```python
from build123d import *

# Parameters (mm, degrees)
F0_W     = 24
F0_H     = 4.9
F0_H_2   = 4.1
F1_DEPTH = 12
F2_DEPTH = 6
F3_DEPTH = 10
F4_SIZE2 = 11.99999
F4_SIZE  = 9.99999
F6_DEPTH = 24
F7_DEPTH = 4
F8_SIZE2 = 1
F8_SIZE  = 8


# Not quite as in the source:
# - a fillet or chamfer is up to 0.001 mm smaller than in the source, because OpenCascade refuses the exact size


with BuildPart() as f1:
    # F0 (on Top) → F1 (new body)
    with BuildSketch(Plane.XY):
        with Locations((-88, -2.45)):
            Rectangle(F0_W, F0_H)
        with Locations((-88, -6.95)):
            Rectangle(F0_W, F0_H_2)
        with Locations((-88, -11.05)):
            Rectangle(F0_W, F0_H_2)
        with Locations((-88, -15.55)):
            Rectangle(F0_W, F0_H)
    extrude(amount=F1_DEPTH)

    # F0 (on Top) → F2 (cut)
    with BuildSketch(Plane.XY):
        with Locations((-88, -6.95)):
            Rectangle(F0_W, F0_H_2)
        with Locations((-88, -11.05)):
            Rectangle(F0_W, F0_H_2)
    extrude(amount=F2_DEPTH, mode=Mode.SUBTRACT)

    # F3 (add): a face of the model
    f3_faces = [f1.faces().sort_by_distance(p)[0] for p in [
        (-88, 0, 6),
    ]]
    extrude(f3_faces, amount=F3_DEPTH)

    # F4 (size 10 and 12 in the source; OpenCascade refuses exactly that, so slightly less here)
    f4_edges = [f1.edges().sort_by_distance(p)[0] for p in [
        (-88, 10, 0),
    ]]
    f4_side = f1.faces().sort_by_distance((-88, 2.55, 0))[0]
    chamfer(f4_edges, length=F4_SIZE, length2=F4_SIZE2, reference=f4_side)

    # F5 (on face) → F6 (join, through all)
    with BuildSketch(Plane.YZ.offset(-76)):
        Polygon((-13.1, 0), (-12.1, 0), (-13.1, 6), align=None)
    extrude(amount=-F6_DEPTH)

    # F7 (add): a face of the model
    f7_faces = [f1.faces().sort_by_distance(p)[0] for p in [
        (-88, -2.449995, 0),
    ]]
    extrude(f7_faces, amount=F7_DEPTH)

    # F8
    f8_edges = [f1.edges().sort_by_distance(p)[0] for p in [
        (-88, -4.9, -4),
    ]]
    f8_side = f1.faces().sort_by_distance((-88, -4.9, 1))[0]
    chamfer(f8_edges, length=F8_SIZE, length2=F8_SIZE2, reference=f8_side)


solid = f1.part
```
The model under review builds one solid part; all positions refer to its coordinate system, in mm. A direction names the side the tool comes from. Round coordinates to 2 decimals unless told otherwise and drop trailing zeros. Loops run counter-clockwise (first coordinate to the right, second up) from the corner with the lowest first, then second, coordinate; pieces in that order, holes last. Notation, with made-up numbers: (34.25, 88) - (56.25, 88) arc R19 cw to (56.25, 109) - close; hole circle Ø11 at (23, 23). An arc over 180 degrees is marked (long way). Write each question's results on one line, items separated by ' | '. Start each with the question number.
Q1. Take a section at C-C on z = 10.5. Give the boundary of the cut face in (x, y), plus the area to 3 significant figures.
Q2. Wall thickness on line 1 along Y through (x, z) = (-83, 1) (3 decimals); line 2 along Z through (x, y) = (-97, -7.25); line 3 along Y through (x, z) = (-91.75, 3.25): over which ranges is each line inside the solid? List them lowest first. Write a range as [from, to].
Q3. Tool access review of faces 4 (the flat face through (-100, -4, 6)), 5 (the flat face through (-88.168, -4.393, -0.056)), 6 (the flat face through (-88, 0, -2)), 7 (the flat face through (-76, -4, 6)), 8 (the flat face through (-88, -15, 0)): name each direction out of +Z, -Z, +X, -X, +Y, -Y from which nothing blocks a thin tool from reaching the whole face with its end or side.
Q4. Take a section at B-B on z = 2.5. Give the boundary of the cut face in (x, y).
Q5. Draft analysis for pull direction Y (two halves, no side actions). For faces 1 (the flat face through (-87.8, -12.6, 3)), 2 (the flat face through (-88, -18, 6)), 3 (the flat face through (-88, -4, 12)), state which applies: pulls with the +Y half, pulls with the -Y half, needs draft (parallel to the pull), parting line crosses it, or undercut.
Q6. Take a section at D-D on y = -9. Give the boundary of the cut face in (x, z), plus the area to 3 significant figures.
Q7. Insertion check: P1, Ø4, axis at x = -91.5, y = -10.5, coming from the -Z side; P2, Ø1.5, axis at x = -95.5, y = 5, coming from the -Z side; P3, Ø2, axis at x = -90, z = 2.5, coming from the +Y side; P4, Ø3, axis at y = -6.5, z = -1, coming from the -X side. Each pin has a flat end and moves straight along its axis. Give the tip position at first contact, or say it passes through.
Data:
1) outline: (-100, -18) - (-76, -18) - (-76, 8.75) - (-100, 8.75) - close | area: 642 mm²
2) line 1: y = [-18, -12.267], [-4.525, 0.833] | line 2: z = [6, 12] | line 3: y = [-18, -12.64], [-4.81, 2.71]
3) face 4: +Z, -Z, -X, +Y, -Y | face 5: -Z, +X, -X | face 6: -Z, +X, -X, +Y | face 7: +Z, -Z, +X, +Y, -Y | face 8: -Z, +X, -X, -Y
4) outline: (-100, -18) - (-76, -18) - (-76, -12.52) - (-100, -12.52) - close; (-100, -4.71) - (-76, -4.71) - (-76, 2.08) - (-100, 2.08) - close
5) face 1: undercut | face 2: pulls with the -Y half | face 3: needs draft
6) outline: (-100, 6) - (-76, 6) - (-76, 12) - (-100, 12) - close | area: 144 mm²
7) P1: stops at z = 0 | P2: stops at z = 5.1 | P3: stops at y = 2.92 | P4: passes through
